Could you check a few things on this model? Use its own coordinates, in mm. A direction names the side the tool comes from. Give positions to 0.01 mm unless a question says otherwise; leave off trailing zeros. Write each question's results on one line, items separated by ' | '. Start each with the question number.
(1) For pin 1 (3 mm diameter, centred on y = 34, z = -27.5, fed in from +X); pin 2 (5.5 mm diameter, centred on x = 25.5, z = -36, fed in from -Y); pin 3 (5.5 mm diameter, centred on x = -24, z = -35, fed in from -Y); pin 4 (3 mm diameter, centred on x = 24, z = -35, fed in from -Y), each with a flat end and sliding along its axis, tell me the tip position at first contact or that it passes through.
(2) If we mould it in two halves opening along X, with no side actions, what happens to faces 1 (the face through (-33.81, 27.14, -27.6)), 2 (the face through (-26.365, 28.726, -32.42)), 3 (the face through (3, 35, -36))? For each: released by +X, released by -X, zero draft, split by the parting line, or undercut.
(3) On a 3-axis mill with a long thin cutter (end or side, diameter ignored), from which of +Z, -Z, +X, -X, +Y, -Y can I reach the whole of each face in a straight line? I mean faces 4 (the face through (-33.82, 34.85, -27.6)), 5 (the face through (26.365, 28.726, -32.42)). Say none if no direction works.
(4) I need wall thicknesses on line 1 (Y direction, x = 25.5, z = -33); line 2 (X direction, y = 31, z = -36); line 3 (Z direction, x = -24, y = 28.6). Which ranges of each line are inside material? Lowest first, please.
(5) Suppose I cut it at A-A (y = 33.5). Count the separate pieces of the cut face and the enclosed holes in it, and give its area (3 significant figures).
from build123d import *

# Parameters (mm, degrees)
BOSS_EXTRU_1_START      = 35
BOSS_EXTRU_1_DEPTH      = 8
CONG_1_R                = 1
ESQUISSE3_R             = 1.75
ENL_V_MAT_EXTRU_1_DEPTH = 56.497932403
ESQUISSE4_R             = 3.5
ENL_V_MAT_EXTRU_2_DEPTH = 3.5
CONG_2_R                = 0.5


with BuildPart() as part:
    # Esquisse1 → Boss.-Extru.1 (new body)
    with BuildSketch(Plane(origin=(0, 0, 0), x_dir=(1, 0, 0), z_dir=(0, 1, 0)).offset(BOSS_EXTRU_1_START)):
        Polygon((0, 40), (30, 40), (38, 15), (0, 15), align=None)
    extrude(amount=-BOSS_EXTRU_1_DEPTH)

    # Esquisse2 → Enlèvement de matière-Révolution1 (revolve, cut)
    with BuildSketch(Plane(origin=(0, 0, 0), x_dir=(0, 0, -1), z_dir=(1, 0, 0))):
        Polygon((39, 0), (27, 115), (-1, 115), (-1, 0), align=None)
    revolve(axis=Axis((0, 115, 1), (0, 1, 0)), mode=Mode.SUBTRACT)

    # Congé1
    cong_1_edges = [part.edges().sort_by_distance(p)[0] for p in [
        (33.101067508, 31.000070332, -15),
        (30, 31, -40),
        (38, 31, -15),
    ]]
    fillet(cong_1_edges, radius=CONG_1_R)

    # Esquisse3 → Enlèv. mat.-Extru.1 (cut, through all)
    with BuildSketch(Plane.XZ.offset(-27)):
        with Locations(Location((24, -35, 0), (0, 0, 270))):
            Circle(ESQUISSE3_R)
    extrude(amount=-ENL_V_MAT_EXTRU_1_DEPTH, mode=Mode.SUBTRACT)

    # Esquisse4 → Enlèv. mat.-Extru.2 (cut)
    with BuildSketch(Plane.XZ.offset(-27)):
        with Locations(Location((24, -35, 0), (0, 0, 270))):
            Circle(ESQUISSE4_R)
    extrude(amount=-ENL_V_MAT_EXTRU_2_DEPTH, mode=Mode.SUBTRACT)

    # Congé2
    cong_2_edges = [part.edges().sort_by_distance(p)[0] for p in [
        (37.437752927, 27, -15.410413589),
        (33.902471767, 27, -27.804775727),
        (29.859634031, 27, -39.807705307),
        (33.664775152, 27, -15.150178589),
        (14.63502381, 35, -40),
        (29.859634031, 35, -39.807705307),
        (33.902471767, 35, -27.804775727),
        (37.437752927, 35, -15.410413589),
        (34.945309997, 35, -15),
        (32.73463145, 35, -15.147278852),
        (14.63502381, 27, -40),
        (19.582003838, 27, -30.60840893),
        (18.969834976, 35, -30.00499673),
        (35.412730047, 27, -15),
    ]]
    fillet(cong_2_edges, radius=CONG_2_R)

    # Symétrie1: part across plane


with BuildPart() as part_1:
    add(part.part)
    add(part.part.mirror(Plane(origin=(0, 27, -40), x_dir=(0, 0, 1), z_dir=(-1, 0, 0))))


solid = part_1.part
Output values:
1) pin 1: x = 34.48 | pin 2: y = 27 | pin 3: y = 30.5 | pin 4: through
2) face 1: released by -X | face 2: undercut | face 3: zero draft
3) face 4: -Z, -X, +Y | face 5: -Y
4) line 1: 30.5 to 35 | line 2: -31.28 to -25.44, -22.56 to 22.56, 25.44 to 31.28 | line 3: -40 to -38.5, -31.5 to -27.18
5) separate pieces: 1 | enclosed holes: 2 | area: 716 mm2
